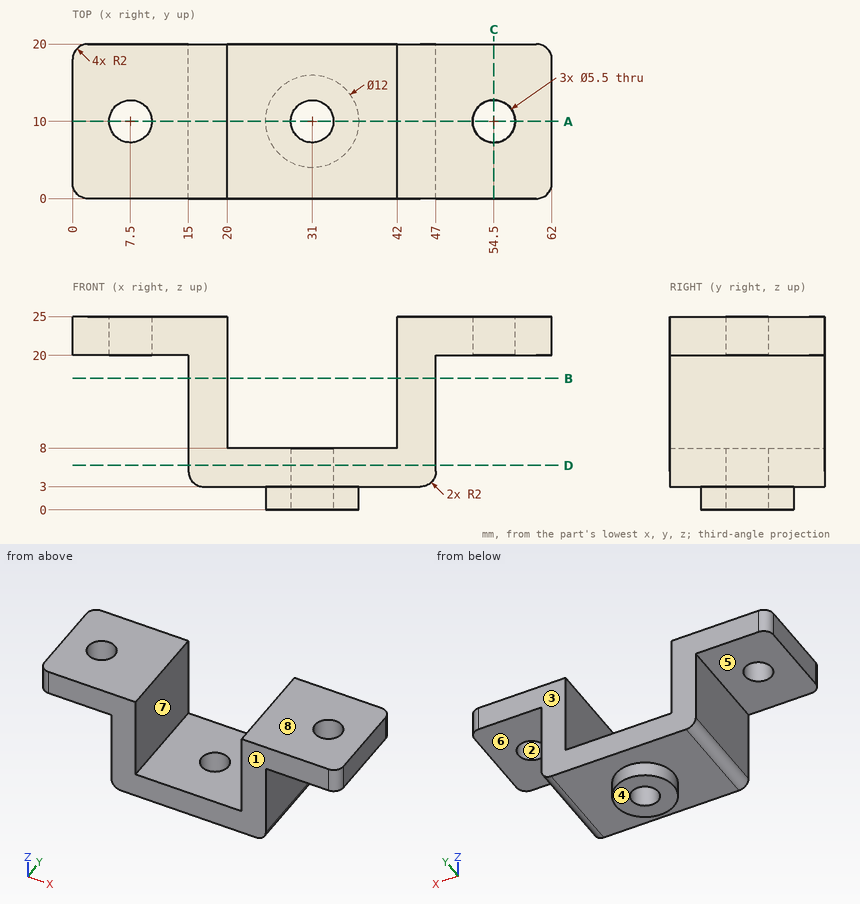
Can you work these out from the drawing? Everything is in mm from the part's minimum corner. A direction names the side the tool comes from. Round coordinates to 2 decimals unless told otherwise and drop trailing zeros. Loops run counter-clockwise (first coordinate to the right, second up) from the corner with the lowest first, then second, coordinate; pieces in that order, holes last. Notation, with made-up numbers: (34, 13) - (55, 13) arc R28 ccw to (55, 45) - close; hole circle Ø7 at (21, 73). An arc over 180 degrees is marked (long way). Answer in a Markdown table with one row per item. Add a question column.
(1) I need wall thicknesses on line 1 along X through (y, z) = (4.25, 18.75); line 2 along Y through (x, z) = (31, 5.25); line 3 along X through (y, z) = (18.5, 6). Which ranges of each line are inside material? Lowest first, please.
(2) For the marked faces 5, 6, 7 and 8, which set-ups out of +Z, -Z, +X, -X, +Y, -Y let a thin tool reach every point of the face, with its end or its side?
(3) If we section it at D-D (z = 5.75): Please give me the cut outline in (x, y).
(4) If we section it at A-A (y = 10): State how many separate pieces and enclosed holes the cut face has, plus the area to 3 significant figures.
(5) If we mould it in two halves opening along Y, with no side actions, what happens to the marked faces 1, 2, 3 and 4? For each: pulls with the +Y half, pulls with the -Y half, needs draft (parallel to the pull), parting line crosses it, or undercut.
(6) If we section it at B-B (z = 17): Please give me the cut outline in (x, y).
(7) If we section it at C-C (x = 54.5): Please give me the cut outline in (y, z).
(8) I'm going to push flat-ended pins straight in: pin 1 (6 mm diameter, centred on x = 30.5, y = 2.5, fed in from +Z); pin 2 (4.5 mm diameter, centred on x = 10, y = 8, fed in from -Z); pin 3 (5 mm diameter, centred on x = 54.5, y = 10, fed in from -Z); pin 4 (4.5 mm diameter, centred on y = 7.5, z = 10, fed in from +X). Where does each tip first touch, or does it pass through?
Model answer:
| question | item | result |
|---|---|---|
| 1 | line 1 | x = 15 to 20, 42 to 47 |
| 1 | line 2 | y = 0 to 7.25, 12.75 to 20 |
| 1 | line 3 | x = 15 to 47 |
| 2 | face 5 | -Z, -X, +Y, -Y |
| 2 | face 6 | -Z, +X, +Y, -Y |
| 2 | face 7 | +Z, +Y, -Y |
| 2 | face 8 | +Z, +X, -X, +Y, -Y |
| 3 | outline | (15, 0) - (47, 0) - (47, 20) - (15, 20) - close; hole circle Ø5.5 at (31, 10) |
| 4 | separate pieces | 4 |
| 4 | enclosed holes | 0 |
| 4 | area | 415 mm² |
| 5 | face 1 | pulls with the -Y half |
| 5 | face 2 | undercut |
| 5 | face 3 | pulls with the +Y half |
| 5 | face 4 | needs draft |
| 6 | outline | (15, 0) - (20, 0) - (20, 20) - (15, 20) - close; (42, 0) - (47, 0) - (47, 20) - (42, 20) - close |
| 7 | outline | (0, 20) - (7.25, 20) - (7.25, 25) - (0, 25) - close; (12.75, 20) - (20, 20) - (20, 25) - (12.75, 25) - close |
| 8 | pin 1 | stops at z = 8 |
| 8 | pin 2 | stops at z = 20 |
| 8 | pin 3 | passes through |
| 8 | pin 4 | stops at x = 47 |
